from build123d import *

# Parameters (mm, degrees)
SKETCH1_R           = 2.5
BOSS_EXTRUDE1_DEPTH = 35
CHAMFER1_SIZE       = 0.5
CUT_EXTRUDE1_DEPTH  = 8


with BuildPart() as part:
    # Sketch1 → Boss-Extrude1 (new body)
    with BuildSketch(Plane.XY):
        Circle(SKETCH1_R)
    extrude(amount=BOSS_EXTRUDE1_DEPTH)

    # Chamfer1
    chamfer1_edges = [part.edges().sort_by_distance(p)[0] for p in [
        (-2.5, 0, 0),
        (-2.5, 0, 35),
    ]]
    chamfer(chamfer1_edges, length=CHAMFER1_SIZE)

    # Sketch2 → Cut-Extrude1 (cut)
    with BuildSketch(Plane.XY.offset(35)):
        Polygon((2, 1.555738269), (2, -1.555738269), (4.460999641, -1.695481282), (5.219104654, -0.46598868), (5.068266404, 0.170018194), (3.416674172, 1.653087335), (3.034604396, 1.88867152), align=None)
        Polygon((-2, 1.555738269), (-2, -1.555738269), (-2.968976112, -3.127221032), (-3.471634936, -2.94714388), (-4.717205701, -1.861261674), (-4.943269872, 1.439275222), align=None)
    cut_extrude1 = extrude(amount=-CUT_EXTRUDE1_DEPTH, mode=Mode.SUBTRACT)

    # Mirror1: Cut-Extrude1 across plane
    add(cut_extrude1.mirror(Plane.XY.offset(17.5)), mode=Mode.SUBTRACT)


solid = part.part
The listing builds one solid part. Answer for the finished solid, in the listing's coordinates (mm). A direction names the side the tool comes from. Round coordinates to 2 decimals unless told otherwise and drop trailing zeros. Order: outer loops, then holes, each group sorted by start corner. A loop starts at its lowest first (then second) coordinate and runs counter-clockwise, first axis right, second up. Notation, with made-up numbers: (18, 66.5) -> (46, 66.5) arc R18 ccw to (46, 86.5) -> close; hole circle Ø5 at (9.25, 87.5). An arc over 180 degrees is marked (long way). Write each question's results on one line, items separated by ' | '. Start each with the question number.
Q1. Straight lines are drawn through the part: probe 1 along Y at (x, z) = (-0.1, 2.5); probe 2 along X at (y, z) = (-1.2, 33.5); probe 3 along X at (y, z) = (-0.3, 18.5). For each, find the intervals that lie inside material, in ascending order. Write a range as from..to.
Q2. Find section B-B (z = 3). Determine the outline of the cut face in (x, y).
Q3. Find section A-A (z = 16). Determine the outline of the cut face in (x, y).
Q4. Which of the six approach directions +Z, -Z, +X, -X, +Y, -Y give full straight-line access (tool end or side, diameter ignored) to faces 1 (the flat face through (2, 0, 31)), 2 (the flat face through (-2, 0, 31)), 3 (the flat face through (-2, 0, 4))?
Q5. Each of these flat-tipped pins is pushed along its axis until it touches: pin 1 (2.5 mm diameter, centred on y = -0.5, z = 5, fed in from +X); pin 2 (0.6 mm diameter, centred on x = 2.5, y = 0.5, fed in from -Z). Where does it stop, or does it pass through?
Worked answers:
1) probe 1: y = -2.5..2.5 | probe 2: x = -2..2 | probe 3: x = -2.48..2.48
2) outline: (-2, -1.5) arc R2.5 ccw to (2, -1.5) -> (2, 1.5) arc R2.5 ccw to (-2, 1.5) -> close
3) outline: circle Ø5 at (0, 0)
4) face 1: +Z, +X, +Y, -Y | face 2: +Z, -X, +Y, -Y | face 3: -Z, -X, +Y, -Y
5) pin 1: stops at x = 2 | pin 2: stops at z = 8
